For this review, take the finished solid that the model builds, in its own axes (mm). A direction names the side the tool comes from. Coordinates: 2 decimals unless noted, no trailing zeros. Write each loop counter-clockwise with the first axis right and the second up, starting at its lowest first coordinate (ties: lowest second). Pieces come first, ordered by that corner, then holes.
1) To check wall thickness, follow line 1 along Y through (x, z) = (50.5, 1.9); line 2 along Y through (x, z) = (-43.9, 4.3); line 3 along X through (y, z) = (-1, 4.55). State the ranges of each line that lie inside material, in increasing order.
2) For faces 1 (the face through (96.75, 20.14, 2.59)), 2 (the face through (-39, 21.6, 3)), 3 (the face through (-30, -22, 3)), 4 (the face through (-33.15, -20, 3)), 5 (the face through (-26, -11, 3)), list the 3-axis set-ups (+Z, -Z, +X, -X, +Y, -Y) from which the entire face can be reached by the end or side of a thin tool; tool diameter is ignored.
3) Mouldability with a two-part tool opening along Y and no side actions: class faces 6 (the face through (-31, -19, 3)), 7 (the face through (-57, 22, 3)), 8 (the face through (-48, -22, 3)) as pulls with the +Y half, pulls with the -Y half, needs draft (parallel to the pull), parting line crosses it, or undercut.
4) We need section B-B on y = -9. Write out the cut boundary in (x, z).
5) We need section C-C on z = 3. Write out the cut boundary in (x, y) (3 decimals).
6) We need section A-A on x = 21. Write out the cut boundary in (y, z), then the cut area to 3 significant figures.
7) Insertion check: P1, Ø2, axis at x = -23, z = 1, coming from the -Y side; P2, Ø2.5, axis at y = -20, z = 2.5, coming from the -X side; P3, Ø1.8, axis at y = -2, z = 2.5, coming from the +X side. Each pin has a flat end and moves straight along its axis. Give the tip position at first contact, or say it passes through.
from build123d import *

# Parameters (mm, degrees)
SKETCH1_R           = 1.5
BOSS_EXTRUDE1_DEPTH = 6
SKETCH2_R           = 1.905
BOSS_EXTRUDE2_DEPTH = 2.54


with BuildPart() as part:
    # Sketch1 → Boss-Extrude1 (new body)
    with BuildSketch(Plane.XY):
        Polygon((0, 0), (100, 0), (100, 44), (0, 44), (-57, 44), (-57, 0), (-51.8, 0), (-51.8, -22), (-44.65, -22), (-44.65, -19), (-48.8, -19), (-48.8, 21.6), (-29, 21.6), (-29, -19), (-33.15, -19), (-33.15, -22), (-26, -22), (-26, 0), align=None)
        with Locations((-43.9, 25.353)):
            Circle(SKETCH1_R, mode=Mode.SUBTRACT)
        with Locations((-33.9, 25.353)):
            Circle(SKETCH1_R, mode=Mode.SUBTRACT)
        with BuildLine():
            Line((0, 2), (98, 2))
            Line((98, 2), (98, 42))
            Line((98, 42), (0, 42))
            ThreePointArc((0, 42), (-20, 22), (0, 2))
        make_face(mode=Mode.SUBTRACT)
    extrude(amount=BOSS_EXTRUDE1_DEPTH)

    # Sketch2 → Boss-Extrude2 (add)
    with BuildSketch(Plane.ZY.offset(-98)):
        with Locations((3, 22)):
            Circle(SKETCH2_R)
    extrude(amount=BOSS_EXTRUDE2_DEPTH)


solid = part.part
Result:
1. line 1: y = 0 to 2, 42 to 44
1. line 2: y = 21.6 to 23.85, 26.85 to 44
1. line 3: x = -51.8 to -48.8, -29 to -26
2. face 1: none
2. face 2: +Z, -Z
2. face 3: +Z, -Z, +X, -X, -Y
2. face 4: +Z, -Z, -Y
2. face 5: +Z, -Z, +X, -Y
3. face 6: undercut
3. face 7: needs draft
3. face 8: pulls with the -Y half
4. outline: (-51.8, 0) - (-48.8, 0) - (-48.8, 6) - (-51.8, 6) - close; (-29, 0) - (-26, 0) - (-26, 6) - (-29, 6) - close
5. outline: (-57, 0) - (-51.8, 0) - (-51.8, -22) - (-44.65, -22) - (-44.65, -19) - (-48.8, -19) - (-48.8, 21.6) - (-29, 21.6) - (-29, -19) - (-33.15, -19) - (-33.15, -22) - (-26, -22) - (-26, 0) - (100, 0) - (100, 44) - (-57, 44) - close; hole circle Ø3 at (-43.9, 25.353); hole circle Ø3 at (-33.9, 25.353); hole (0, 2) - (98, 2) - (98, 20.095) - (95.46, 20.095) - (95.46, 23.905) - (98, 23.905) - (98, 42) - (0, 42) arc R20 ccw to start
6. outline: (0, 0) - (2, 0) - (2, 6) - (0, 6) - close; (42, 0) - (44, 0) - (44, 6) - (42, 6) - close
6. area: 24.0 mm2
7. P1: stops at y = 0
7. P2: stops at x = -51.8
7. P3: stops at x = -26
